```python
from build123d import *

# Parameters (mm, degrees)
SKETCH1_W           = 32
SKETCH1_H           = 26
SKETCH1_R           = 1.25
SKETCH1_W_2         = 26
SKETCH1_H_2         = 13
BOSS_EXTRUDE1_DEPTH = 5
FILLET1_R           = 3


with BuildPart() as part:
    # Sketch1 → Boss-Extrude1 (new body)
    with BuildSketch(Plane(origin=(0, 0, 0), x_dir=(1, 0, 0), z_dir=(0, 1, 0))):
        with Locations((16, 13)):
            Rectangle(SKETCH1_W, SKETCH1_H)
        with Locations((3, 21)):
            Circle(SKETCH1_R, mode=Mode.SUBTRACT)
        with Locations((29, 21)):
            Circle(SKETCH1_R, mode=Mode.SUBTRACT)
        with Locations((16, 9.5)):
            Rectangle(SKETCH1_W_2, SKETCH1_H_2, mode=Mode.SUBTRACT)
    extrude(amount=BOSS_EXTRUDE1_DEPTH)

    # Fillet1
    fillet1_edges = [part.edges().sort_by_distance(p)[0] for p in [
        (0, 2.5, -26),
        (32, 2.5, -26),
        (32, 2.5, 0),
        (0, 2.5, 0),
    ]]
    fillet(fillet1_edges, radius=FILLET1_R)


solid = part.part
```
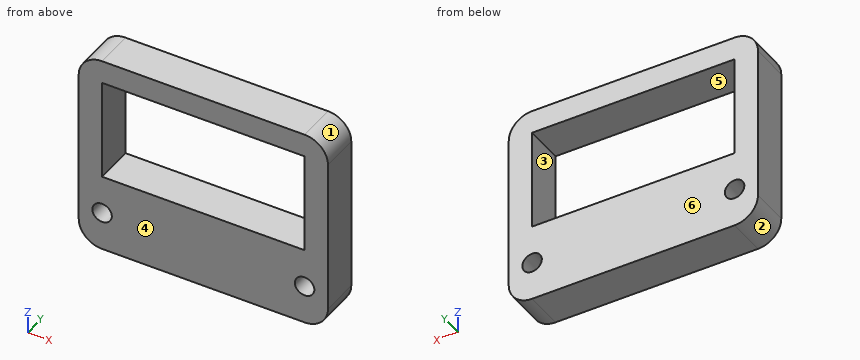
Model file for the job. Use its own axes, mm. Face numbers are marked on the shaded views. A direction names the side the tool comes from. Coordinates: 2 decimals unless noted, no trailing zeros. Loops run counter-clockwise (first coordinate to the right, second up) from the corner with the lowest first, then second, coordinate; pieces in that order, holes last. Notation, with made-up numbers: (88.25, -0.75) - (98.25, -0.75) arc R32 cw to (98.25, 38.25) - close; hole circle Ø9 at (39.5, -16). An arc over 180 degrees is marked (long way). Answer as a JSON object with one key per item and string values. Group by question number.
(1) Tool access for the marked faces 5 and 6: list every direction of +Z, -Z, +X, -X, +Y, -Y with a clear straight run to the whole face (end or side of a thin tool).
(2) Two-plate mould, pull along X, no slides. Class the marked faces 1, 2, 3 and 4: released by +X, released by -X, zero draft, split by the parting line, or undercut.
(3) Cut at A-A (x = 8). Give the cut face in (y, z).
(4) Cut at C-C (y = 0.9). Give the cut face in (x, z).
(5) Cut at B-B (z = -3.5). Give the cut face in (x, y).
(6) Probe line 1 along X through (y, z) = (2.5, -21); line 2 along X through (y, z) = (4.2, -13.25); line 3 along Z through (x, y) = (28, 2.4). List the from-to ranges inside material, lowest first.
(7) Cut at D-D (z = -21). Give the cut face in (x, y), then the cut area to 3 significant figures.
Geometry says:
{
 "1": {"face 5": "+Y, -Y", "face 6": "+Z, -Z, +X, -X, +Y"},
 "2": {"face 1": "released by +X", "face 2": "released by -X", "face 3": "undercut", "face 4": "zero draft"},
 "3": {"outline": "(0, -26) - (5, -26) - (5, -16) - (0, -16) - close; (0, -3) - (5, -3) - (5, 0) - (0, 0) - close"},
 "4": {"outline": "(0, -23) arc R3 ccw to (3, -26) - (29, -26) arc R3 ccw to (32, -23) - (32, -3) arc R3 ccw to (29, 0) - (3, 0) arc R3 ccw to (0, -3) - close; hole circle Ø2.5 at (3, -21); hole (3, -16) - (29, -16) - (29, -3) - (3, -3) - close; hole circle Ø2.5 at (29, -21)"},
 "5": {"outline": "(0, 0) - (3, 0) - (3, 5) - (0, 5) - close; (29, 0) - (32, 0) - (32, 5) - (29, 5) - close"},
 "6": {"line 1": "x = 0 to 1.75, 4.25 to 27.75, 30.25 to 32", "line 2": "x = 0 to 3, 29 to 32", "line 3": "z = -26 to -21.75, -20.25 to -16, -3 to 0"},
 "7": {"outline": "(0, 0) - (1.75, 0) - (1.75, 5) - (0, 5) - close; (4.25, 0) - (27.75, 0) - (27.75, 5) - (4.25, 5) - close; (30.25, 0) - (32, 0) - (32, 5) - (30.25, 5) - close", "area": "135 mm^2"}
}
